For this review, use the dimensioned drawing (mm, ordinates from the lowest corner) and the shaded views. Coordinates: 2 decimals unless noted, no trailing zeros. Write each loop counter-clockwise with the first axis right and the second up, starting at its lowest first coordinate (ties: lowest second). Pieces come first, ordered by that corner, then holes. Notation, with made-up numbers: (53.25, -2.5) - (71.25, -2.5) arc R34 ccw to (71.25, 31.5) - close; hole circle Ø8 at (-36, 68.25). An arc over 180 degrees is marked (long way). Answer as a JSON object with one key per item and string values.
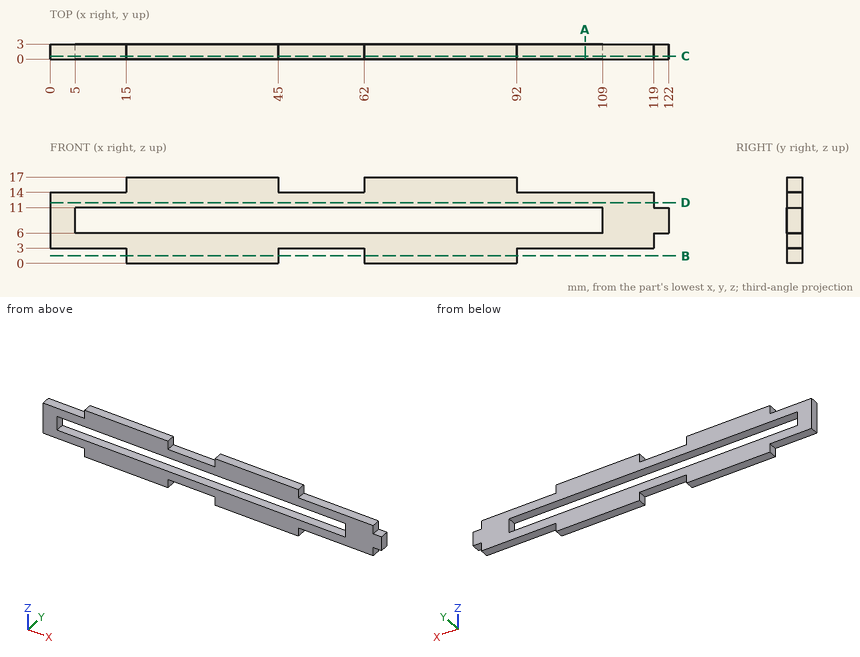
(1) Take a section at D-D, the plane z = 12. Write out the cut boundary in (x, y), and give its area (3 significant figures).
Solved:
{"outline": "(0, 0) - (119, 0) - (119, 3) - (0, 3) - close", "area": "357 mm^2"}
(2) Take a section at B-B, the plane z = 1.5. Write out the cut boundary in (x, y).
Solved:
{"outline": "(15, 0) - (45, 0) - (45, 3) - (15, 3) - close; (62, 0) - (92, 0) - (92, 3) - (62, 3) - close"}
(3) Take a section at C-C, the plane y = 0.6. Write out the cut boundary in (x, z), and give its area (3 significant figures).
Solved:
{"outline": "(0, 3) - (15, 3) - (15, 0) - (45, 0) - (45, 3) - (62, 3) - (62, 0) - (92, 0) - (92, 3) - (119, 3) - (119, 6) - (122, 6) - (122, 11) - (119, 11) - (119, 14) - (92, 14) - (92, 17) - (62, 17) - (62, 14) - (45, 14) - (45, 17) - (15, 17) - (15, 14) - (0, 14) - close; hole (5, 6) - (109, 6) - (109, 11) - (5, 11) - close", "area": "1,160 mm^2"}
(4) To check wall thickness, follow line 1 (Z direction, x = 77.5, y = 2.75); line 2 (X direction, y = 0.85, z = 0.75); line 3 (Z direction, x = 106, y = 1.65). State the ranges of each line that lie inside material, in increasing order. Write a range as from..to.
Solved:
{"line 1": "z = 0..6, 11..17", "line 2": "x = 15..45, 62..92", "line 3": "z = 3..6, 11..14"}
(5) Take a section at A-A, the plane x = 105.5. Write out the cut boundary in (y, z).
Solved:
{"outline": "(0, 3) - (3, 3) - (3, 6) - (0, 6) - close; (0, 11) - (3, 11) - (3, 14) - (0, 14) - close"}
(6) For pin 1 (1.5 mm diameter, centred on y = 1.5, z = 15, fed in from -X); pin 2 (1.5 mm diameter, centred on y = 2, z = 8.5, fed in from -X); pin 3 (0.9 mm diameter, centred on x = 120, y = 1.5, fed in from -Z); pin 4 (1.5 mm diameter, centred on x = 121, y = 1, fed in from +Z), all flat-tipped, find the tip position at first contact; note any pin that passes through.
Solved:
{"pin 1": "stops at x = 15", "pin 2": "stops at x = 0", "pin 3": "stops at z = 6", "pin 4": "stops at z = 11"}
